The model under review builds one solid part; all positions refer to its coordinate system, in mm. Face numbers are marked on the shaded views. A direction names the side the tool comes from. Round coordinates to 2 decimals unless told otherwise and drop trailing zeros. Loops run counter-clockwise (first coordinate to the right, second up) from the corner with the lowest first, then second, coordinate; pieces in that order, holes last. Notation, with made-up numbers: M 55.25,52 L 112.25,52 A19 ccw 112.25,60 Z; hole C -17,54.5 d1. An arc over 180 degrees is marked long. Return JSON: item names as keys, results as strings. Group by question number.
Q1. Consider section A-A (y = 21.15). State the section outline as (x, z) points.
Q2. For the marked faces 1, 2 and 3, list the 3-axis set-ups (+Z, -Z, +X, -X, +Y, -Y) from which the entire face can be reached by the end or side of a thin tool; tool diameter is ignored.
Q3. To check wall thickness, follow line 1 along Y through (x, z) = (36.65, 5.75); line 2 along Y through (x, z) = (21.15, 4). State the ranges of each line that lie inside material, in increasing order.
Q4. Clearance check with flat-ended pins moving along their axes: pin 1 Ø2.5 at (x, y) = (36.65, 5.65) entering from +Z; pin 2 Ø5 at (x, y) = (5.65, 5.65) entering from +Z; pin 3 Ø5 at (x, y) = (5.65, 36.65) entering from -Z. State where each tip first meets the part, or that it passes through.
Q5. Consider section C-C (z = 4). State the section outline as (x, y) points, and give its area (3 significant figures).
Q6. Draft analysis for pull direction X (two halves, no side actions). For the marked faces 4, 5 and 6, state which applies: pulls with the +X half, pulls with the -X half, needs draft (parallel to the pull), parting line crosses it, or undercut.
Q7. Consider section D-D (x = 5.65). State the section outline as (y, z) points, and give its area (3 significant figures).
from build123d import *

# Parameters (mm, degrees)
ESQUISSE1_W             = 42.3
ESQUISSE1_H             = 42.3
BOSS_EXTRU_1_DEPTH      = 16
ESQUISSE2_R             = 1.5
ENL_V_MAT_EXTRU_2_DEPTH = 62.92398566
CONG_1_R                = 3
CONG_2_R                = 3
ESQUISSE4_R             = 11.5
ENL_V_MAT_EXTRU_4_DEPTH = 62.92398566
ESQUISSE5_R             = 2.85
ENL_V_MAT_EXTRU_5_DEPTH = 10
ESQUISSE6_R             = 4.35
ENL_V_MAT_EXTRU_6_DEPTH = 12
ESQUISSE7_R             = 14.5
ENL_V_MAT_EXTRU_7_DEPTH = 2


with BuildPart() as part:
    # Esquisse1 → Boss.-Extru.1 (new body)
    with BuildSketch(Plane.XY):
        with Locations((21.15, 21.15)):
            Rectangle(ESQUISSE1_W, ESQUISSE1_H)
    extrude(amount=BOSS_EXTRU_1_DEPTH)

    # Esquisse2 → Enlèv. mat.-Extru.2 (cut, through all)
    with BuildSketch(Plane.XY):
        with Locations((36.65, 36.65)):
            Circle(ESQUISSE2_R)
        with Locations((5.65, 36.65)):
            Circle(ESQUISSE2_R)
        with Locations((5.65, 5.65)):
            Circle(ESQUISSE2_R)
        with Locations((36.65, 5.65)):
            Circle(ESQUISSE2_R)
    extrude(amount=ENL_V_MAT_EXTRU_2_DEPTH, mode=Mode.SUBTRACT)

    # Congé1
    cong_1_edges = [part.edges().sort_by_distance(p)[0] for p in [
        (0, 42.3, 8),
        (42.3, 42.3, 8),
    ]]
    fillet(cong_1_edges, radius=CONG_1_R)

    # Congé2
    cong_2_edges = [part.edges().sort_by_distance(p)[0] for p in [
        (42.3, 0, 8),
        (0, 0, 8),
    ]]
    fillet(cong_2_edges, radius=CONG_2_R)

    # Esquisse4 → Enlèv. mat.-Extru.4 (cut, through all)
    with BuildSketch(Plane.XY):
        with Locations((21.15, 21.15)):
            Circle(ESQUISSE4_R)
    extrude(amount=ENL_V_MAT_EXTRU_4_DEPTH, mode=Mode.SUBTRACT)

    # Esquisse5 → Enlèv. mat.-Extru.5 (cut)
    with BuildSketch(Plane.XY):
        with Locations((36.65, 36.65)):
            Circle(ESQUISSE5_R)
        with Locations((5.65, 36.65)):
            Circle(ESQUISSE5_R)
        with Locations((5.65, 5.65)):
            Circle(ESQUISSE5_R)
        with Locations((36.65, 5.65)):
            Circle(ESQUISSE5_R)
    extrude(amount=ENL_V_MAT_EXTRU_5_DEPTH, mode=Mode.SUBTRACT)

    # Esquisse6 → Enlèv. mat.-Extru.6 (cut)
    with BuildSketch(Plane.XY):
        with Locations((29.3, 6.5)):
            Circle(ESQUISSE6_R)
        with Locations((13, 6.5)):
            Circle(ESQUISSE6_R)
    extrude(amount=ENL_V_MAT_EXTRU_6_DEPTH, mode=Mode.SUBTRACT)

    # Esquisse7 → Enlèv. mat.-Extru.7 (cut)
    with BuildSketch(Plane.XY.offset(16)):
        with Locations((21.15, 21.15)):
            Circle(ESQUISSE7_R)
    extrude(amount=-ENL_V_MAT_EXTRU_7_DEPTH, mode=Mode.SUBTRACT)


solid = part.part
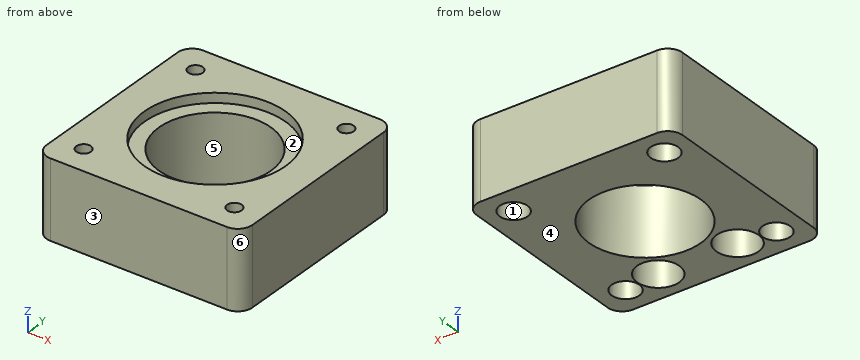
Values:
{
 "1": {"outline": "M 0,0 L 9.65,0 L 9.65,14 L 6.65,14 L 6.65,16 L 0,16 Z; M 32.65,0 L 42.3,0 L 42.3,16 L 35.65,16 L 35.65,14 L 32.65,14 Z"},
 "2": {"face 1": "-Z", "face 2": "+Z", "face 3": "+Z, -Z, +X, -X, -Y"},
 "3": {"line 1": "y = 0 to 2.8, 8.5 to 33.8, 39.5 to 42.3", "line 2": "y = 0 to 9.65, 32.65 to 42.3"},
 "4": {"pin 1": "passes through", "pin 2": "stops at z = 16", "pin 3": "stops at z = 10"},
 "5": {"outline": "M 0,3 A3 ccw 3,0 L 39.3,0 A3 ccw 42.3,3 L 42.3,39.3 A3 ccw 39.3,42.3 L 3,42.3 A3 ccw 0,39.3 Z; hole C 5.65,5.65 d5.7; hole C 5.65,36.65 d5.7; hole C 13,6.5 d8.7; hole C 21.15,21.15 d23; hole C 29.3,6.5 d8.7; hole C 36.65,5.65 d5.7; hole C 36.65,36.65 d5.7", "area": "1,150 mm2"},
 "6": {"face 4": "needs draft", "face 5": "undercut", "face 6": "pulls with the +X half"},
 "7": {"outline": "M 0,0 L 2.8,0 L 2.8,10 L 4.15,10 L 4.15,16 L 0,16 Z; M 7.15,10 L 8.5,10 L 8.5,0 L 33.8,0 L 33.8,10 L 35.15,10 L 35.15,16 L 7.15,16 Z; M 38.15,10 L 39.5,10 L 39.5,0 L 42.3,0 L 42.3,16 L 38.15,16 Z", "area": "527 mm2"}
}
